Geometry: final body of the model. Coordinates: model frame, mm. A direction names the side the tool comes from. Give positions to 0.01 mm unless a question says otherwise; leave off trailing zeros. Order: outer loops, then holes, each group sorted by start corner. A loop starts at its lowest first (then second) coordinate and runs counter-clockwise, first axis right, second up. Notation, with made-up numbers: (69, 36.5) -> (76, 36.5) arc R16 cw to (76, 57.5) -> close; hole circle Ø5 at (-30, -19). An arc over 180 degrees is marked (long way). One line per question, with ' | ' between items. Start each with the question number.
(1) First-contact query: pin 1 Ø1 at (x, y) = (28, 12.5) entering from +Z; pin 2 Ø2.5 at (y, z) = (1.5, 18.5) entering from -X; pin 3 Ø0.9 at (y, z) = (2, 14.5) entering from -X. Flat tips, straight axial feed; report the tip coordinate or a pass-through.
(2) Section A-A (z = 23). Return loops of the section in (x, y).
(3) Section D-D (x = 17.47). Return loops of the section in (y, z), then the cut area to 3 significant figures.
(4) Section B-B (y = 18.45). Return loops of the section in (x, z).
(5) Section C-C (x = 28.85). Return loops of the section in (y, z).
(6) Ray query, L1, parallel to Y at x = 4.3, z = 28.7; L2, parallel to Z at x = 3.5, y = 17.5; L3, parallel to X at y = 9, z = 23.5. Return the intervals inside material, ascending.
(7) Set-up query: faces 1 (the face through (4, 11, 10)), 2 (the face through (49.1, 13, 17)), 3 (the face through (3.823, 6.402, 29.035)), 4 (the face through (42.73, 2, 17)). Return all of +Z, -Z, +X, -X, +Y, -Y with unobstructed straight access to the full face (end or side cutting, diameter ignored); none if empty.
(8) Mould query, pull axis Y, two halves, no side actions, for faces 5 (the face through (4, 19, 5)), 6 (the face through (7.7, 26.14, 23.64)), 7 (the face through (53, 9, 26.5)). Classes: +Y half, -Y half, draft (parallel to the pull), parting line (faces both ways), or undercut.
```python
from build123d import *

# Parameters (mm, degrees)
BOSS_EXTRUDE1_DEPTH = 27
SKETCH2_R           = 2.2
CUT_EXTRUDE1_DEPTH  = 5
SKETCH4_W           = 40.5
SKETCH4_H           = 21
CUT_EXTRUDE2_DEPTH  = 28.5
SKETCH5_W           = 40.5
SKETCH5_H           = 3
CUT_EXTRUDE4_DEPTH  = 28.5
CUT_EXTRUDE7_DEPTH  = 3
SKETCH6_W           = 10
SKETCH6_H           = 16
CUT_EXTRUDE5_DEPTH  = 28.5
FILLET1_R           = 3
FILLET2_R           = 1
SKETCH9_R           = 3.05
CUT_EXTRUDE6_DEPTH  = 10


with BuildPart() as part:
    # Sketch1 → Boss-Extrude1 (new body)
    with BuildSketch(Plane(origin=(0, 0, 0), x_dir=(1, 0, 0), z_dir=(0, 1, 0))):
        Polygon((0, 0), (60, 0), (60, -31.5), (0, -31.5), (0, -26.5), (0, -3), align=None)
    extrude(amount=BOSS_EXTRUDE1_DEPTH)

    # Sketch2 → Cut-Extrude1 (cut)
    with BuildSketch(Plane.XY.offset(31.5)):
        with Locations((4.3, 18.45)):
            Circle(SKETCH2_R)
        with Locations((4.3, 8.55)):
            Circle(SKETCH2_R)
        with Locations((53.4, 18.45)):
            Circle(SKETCH2_R)
        with Locations((53.4, 8.55)):
            Circle(SKETCH2_R)
    extrude(amount=-CUT_EXTRUDE1_DEPTH, mode=Mode.SUBTRACT)

    # Sketch4 → Cut-Extrude2 (cut)
    with BuildSketch(Plane.XY.offset(31.5)):
        with Locations((28.85, 13.5)):
            Rectangle(SKETCH4_W, SKETCH4_H)
    extrude(amount=-CUT_EXTRUDE2_DEPTH, mode=Mode.SUBTRACT)

    # Sketch5 → Cut-Extrude4 (cut)
    with BuildSketch(Plane.XY.offset(31.5)):
        with Locations((28.85, 25.5)):
            Rectangle(SKETCH5_W, SKETCH5_H)
    extrude(amount=-CUT_EXTRUDE4_DEPTH, mode=Mode.SUBTRACT)

    # Sketch10 → Cut-Extrude7 (cut)
    with BuildSketch(Plane(origin=(0, 3, 0), x_dir=(1, 0, 0), z_dir=(0, 1, 0))):
        with BuildLine():
            Line((31.35, -26.25), (31.35, -8.25))
            ThreePointArc((31.35, -8.25), (28.85, -5.75), (26.35, -8.25))
            Line((26.35, -8.25), (26.35, -26.25))
            ThreePointArc((26.35, -26.25), (28.85, -28.75), (31.35, -26.25))
        make_face()
        with BuildLine():
            Line((42.73, -26.25), (42.73, -8.25))
            ThreePointArc((42.73, -8.25), (40.23, -5.75), (37.73, -8.25))
            Line((37.73, -8.25), (37.73, -26.25))
            ThreePointArc((37.73, -26.25), (40.23, -28.75), (42.73, -26.25))
        make_face()
        with BuildLine():
            Line((19.97, -26.25), (19.97, -8.25))
            ThreePointArc((19.97, -8.25), (17.47, -5.75), (14.97, -8.25))
            Line((14.97, -8.25), (14.97, -26.25))
            ThreePointArc((14.97, -26.25), (17.47, -28.75), (19.97, -26.25))
        make_face()
    extrude(amount=-CUT_EXTRUDE7_DEPTH, mode=Mode.SUBTRACT)

    # Sketch6 → Cut-Extrude5 (cut)
    with BuildSketch(Plane(origin=(8.6, 0, 0), x_dir=(0, 0, -1), z_dir=(1, 0, 0))):
        with Locations((-10, 19)):
            Rectangle(SKETCH6_W, SKETCH6_H)
    extrude(amount=-CUT_EXTRUDE5_DEPTH, mode=Mode.SUBTRACT)

    # Fillet1
    fillet1_edges = [part.edges().sort_by_distance(p)[0] for p in [
        (8.6, 27, 23.25),
        (0, 27, 23.25),
        (0, 27, 2.5),
        (8.6, 27, 4),
        (49.1, 27, 17.25),
        (0, 0, 15.75),
    ]]
    fillet(fillet1_edges, radius=FILLET1_R)

    # Fillet2
    fillet2_edges = [part.edges().sort_by_distance(p)[0] for p in [
        (4.3, 11, 15),
        (0, 17.5, 5),
        (0, 11, 10),
        (4.3, 11, 5),
        (8.6, 11, 10),
        (8.6, 17.5, 5),
        (0, 17.5, 15),
        (4.3, 27, 5),
        (7.721320344, 26.121320344, 5),
        (0.878679656, 26.121320344, 5),
        (8.6, 17.5, 15),
        (4.3, 27, 15),
        (7.721320344, 26.121320344, 15),
        (0.878679656, 26.121320344, 15),
    ]]
    fillet(fillet2_edges, radius=FILLET2_R)

    # Sketch9 → Cut-Extrude6 (cut)
    with BuildSketch(Plane(origin=(0, 0, 0), x_dir=(-1, 0, 0), z_dir=(0, 0, -1))):
        with Locations((-17.68, 12)):
            Circle(SKETCH9_R)
    extrude(amount=-CUT_EXTRUDE6_DEPTH, mode=Mode.SUBTRACT)


solid = part.part
```
Response:
1) pin 1: stops at z = 3 | pin 2: stops at x = 0.01 | pin 3: stops at x = 0.05
2) outline: (0, 3) arc R3 ccw to (3, 0) -> (14.97, 0) -> (14.97, 3) -> (8.6, 3) -> (8.6, 24) arc R3 ccw to (5.6, 27) -> (3, 27) arc R3 ccw to (0, 24) -> close; (19.97, 0) -> (26.35, 0) -> (26.35, 3) -> (19.97, 3) -> close; (31.35, 0) -> (37.73, 0) -> (37.73, 3) -> (31.35, 3) -> close; (42.73, 0) -> (60, 0) -> (60, 27) -> (52.1, 27) arc R3 ccw to (49.1, 24) -> (49.1, 3) -> (42.73, 3) -> close
3) outline: (0, 0) -> (8.96, 0) -> (8.96, 3) -> (3, 3) -> (3, 5.75) -> (0, 5.75) -> close; (0, 28.75) -> (3, 28.75) -> (3, 31.5) -> (0, 31.5) -> close; (15.04, 0) -> (27, 0) -> (27, 3) -> (15.04, 3) -> close | area: 79.2 mm^2
4) outline: (0, 0) -> (60, 0) -> (60, 31.5) -> (55.6, 31.5) -> (55.6, 26.5) -> (51.2, 26.5) -> (51.2, 31.5) -> (49.1, 31.5) -> (49.1, 3) -> (8.6, 3) -> (8.6, 4) arc R1 ccw to (7.6, 5) -> (1, 5) arc R1 ccw to (0, 4) -> close; (0, 16) arc R1 ccw to (1, 15) -> (7.6, 15) arc R1 ccw to (8.6, 16) -> (8.6, 31.5) -> (6.5, 31.5) -> (6.5, 26.5) -> (2.1, 26.5) -> (2.1, 31.5) -> (0, 31.5) -> close
5) outline: (0, 0) -> (27, 0) -> (27, 3) -> (3, 3) -> (3, 5.75) -> (0, 5.75) -> close; (0, 28.75) -> (3, 28.75) -> (3, 31.5) -> (0, 31.5) -> close
6) L1: y = 0 to 6.35, 10.75 to 16.25, 20.65 to 27 | L2: z = 0 to 5, 15 to 26.5 | L3: x = 0 to 8.6, 49.1 to 60
7) face 1: -X, +Y | face 2: +Z, +Y | face 3: +Z | face 4: +Y, -Y
8) face 5: draft | face 6: +Y half | face 7: undercut
